Could you check a few things on this drawing? It's one solid part, dimensions in mm from its lowest x, y, z. A direction names the side the tool comes from. Give positions to 0.01 mm unless a question says otherwise; leave off trailing zeros. Write each loop counter-clockwise with the first axis right and the second up, starting at its lowest first coordinate (ties: lowest second). Pieces come first, ordered by that corner, then holes.
1. I'm going to push flat-ended pins straight in: pin 1 (0.9 mm diameter, centred on y = 13.5, z = 23.5, fed in from +X); pin 2 (2.5 mm diameter, centred on x = 8, z = 23.5, fed in from +Y); pin 3 (0.9 mm diameter, centred on y = 15, z = 24.5, fed in from -X). Where does each tip first touch, or does it pass through?
2. Suppose I cut it at C-C (z = 12.75). Please give me the cut outline in (x, y).
3. Suppose I cut it at B-B (y = 12.5). Please give me the cut outline in (x, z).
4. Suppose I cut it at D-D (z = 7). Please give me the cut outline in (x, y).
5. On a 3-axis mill with a long thin cutter (end or side, diameter ignored), from which of +Z, -Z, +X, -X, +Y, -Y can I reach the whole of each face in a straight line? I mean the marked faces 1, 2 and 3. Say none if no direction works.
6. If I drill on probe 1 along X at (y, z) = (15, 13.75); probe 2 along Z at (x, y) = (3, 18.75); probe 3 along Z at (x, y) = (9, 15), over which ranges is the centre line in solid material (lowest first)?
7. Suppose I cut it at A-A (x = 8). Please give me the cut outline in (y, z), and give its area (4 significant figures).
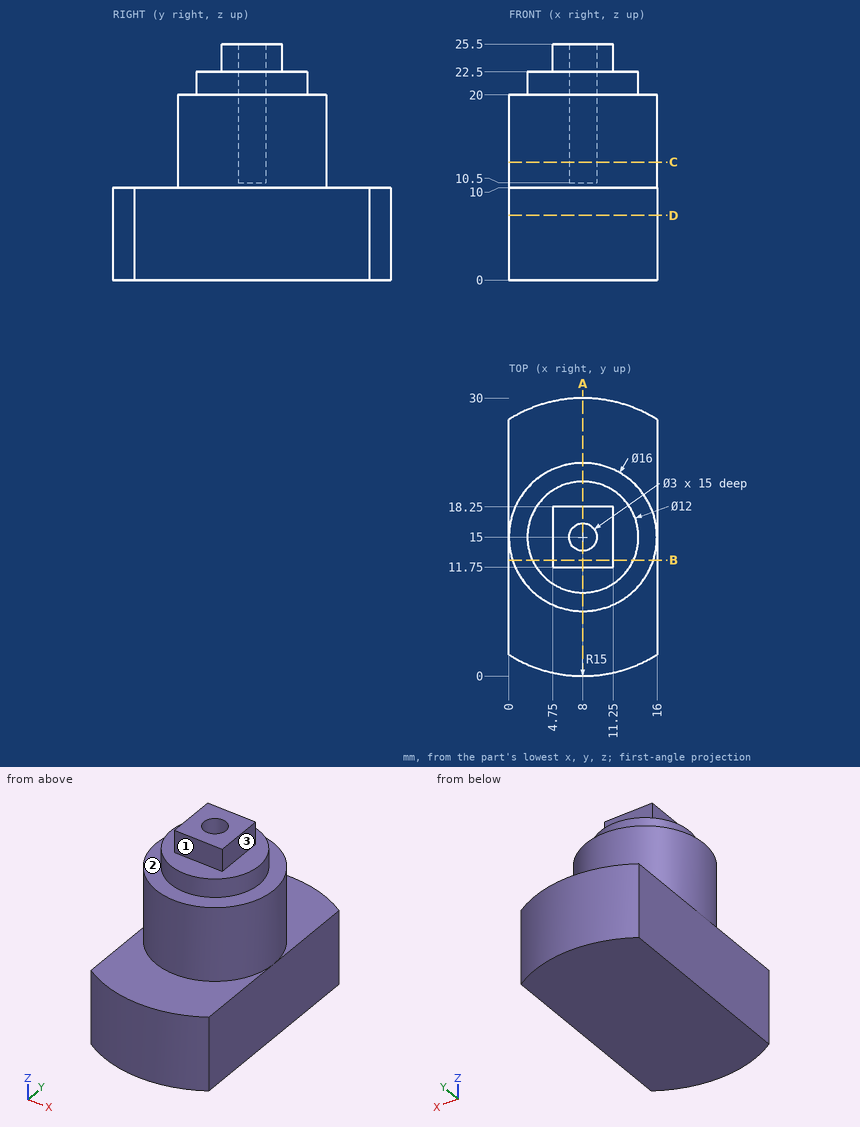
Checks:
1. pin 1: stops at x = 11.25
1. pin 2: stops at y = 21
1. pin 3: stops at x = 4.75
2. outline: circle Ø16 at (8, 15); hole circle Ø3 at (8, 15)
3. outline: (0, 0) - (16, 0) - (16, 10) - (15.6, 10) - (15.6, 20) - (13.45, 20) - (13.45, 22.5) - (11.25, 22.5) - (11.25, 25.5) - (4.75, 25.5) - (4.75, 22.5) - (2.55, 22.5) - (2.55, 20) - (0.4, 20) - (0.4, 10) - (0, 10) - close
4. outline: (0, 2.31) arc R15 ccw to (16, 2.31) - (16, 27.69) arc R15 ccw to (0, 27.69) - close
5. face 1: +Z, +X, -X, -Y
5. face 2: +Z
5. face 3: +Z, +X, +Y, -Y
6. probe 1: x = 0 to 6.5, 9.5 to 16
6. probe 2: z = 0 to 20
6. probe 3: z = 0 to 10.5
7. outline: (0, 0) - (30, 0) - (30, 10) - (23, 10) - (23, 20) - (21, 20) - (21, 22.5) - (18.25, 22.5) - (18.25, 25.5) - (16.5, 25.5) - (16.5, 10.5) - (13.5, 10.5) - (13.5, 25.5) - (11.75, 25.5) - (11.75, 22.5) - (9, 22.5) - (9, 20) - (7, 20) - (7, 10) - (0, 10) - close
7. area: 464.5 mm2
